Design review of the part built by this model. Coordinates are the model's own, in mm. A direction names the side the tool comes from. Coordinates: 2 decimals unless noted, no trailing zeros. Loops run counter-clockwise (first coordinate to the right, second up) from the corner with the lowest first, then second, coordinate; pieces in that order, holes last. Notation, with made-up numbers: (30, 16.5) - (85, 16.5) arc R13 ccw to (85, 25.5) - close; hole circle Ø7 at (48, 29). An arc over 180 degrees is marked (long way). Use one line per item in the form item = value. Start each with the question number.
(1) Add section D-D (z = 1.9). State the section outline as (x, y) points, plus the area to 3 significant figures.
(2) Add section B-B (z = 0.85). Count the separate pieces of the cut face and the enclosed holes in it, plus the area to 3 significant figures.
(3) The part is to be moulded in two halves that separate along Y. For faces 3 (the face through (-1, -0.29, 2)), 4 (the face through (0, 7.736, 1)), say which applies: pulls with the +Y half, pulls with the -Y half, needs draft (parallel to the pull), parting line crosses it, or undercut.
(4) Clearance check with flat-ended pins moving along their axes: pin 1 Ø1 at (x, z) = (-1.5, 2) entering from -Y; pin 2 Ø1.4 at (x, y) = (-2.53, 6.36) entering from +Z; pin 3 Ø2.5 at (x, y) = (-6.95, -1.31) entering from +Z. State where each tip first meets the part, or that it passes through.
(5) For L1, parallel to Y at x = 7, z = 0.6; L2, parallel to Y at x = -2.5, z = 0.75; L3, parallel to Y at x = -2.75, z = 1.3, list the stretches that pass through material, from the lowest coordinate up.
(6) Tool access review of faces 1 (the face through (-2.2, 1, 2)), 2 (the face through (-8.65, 7.45, 0.81)): name each direction out of +Z, -Z, +X, -X, +Y, -Y from which nothing blocks a thin tool from reaching the whole face with its end or side.
(7) Add section C-C (y = -1). State the section outline as (x, z) points, plus the area to 3 significant figures.
Autodesk Fusion 360 part; units mm, degrees
sketch "Sketch2" plane through (0, 0, 0) normal (0, 0, 1) x (1, 0, 0)
  line L0 (-8.9478, 7.7363) -> (9.0022, 7.7363)
  line L1 (9.0022, 7.7363) -> (9.0022, -5.5137)
  line L2 (9.0022, -5.5137) -> (-8.9478, -5.5137)
  line L3 (-8.9478, -5.5137) -> (-8.9478, 7.7363)
  line L4 (-8.9478, 7.7363) -> (9.0022, -5.5137) construction
  line L5 (-8.9478, -5.5137) -> (9.0022, 7.7363) construction
  line L6 (-9.5685, 6.7363) -> (10, 6.7363) construction
  line L7 (-9.5685, 6.3613) -> (10, 6.3613) construction
  line L8 (-10.5, -4.5137) -> (10.5, -4.5137) construction
  line L9 (-10.5, -4.1387) -> (10.5, -4.1387) construction
  line L10 (8.5022, 9) -> (8.5022, -6.5) construction
  line L11 (7.0022, 9) -> (7.0022, -6.5) construction
  line L12 (-8.4478, 9.5) -> (-8.4478, -7) construction
  line L13 (-6.9478, 9.5) -> (-6.9478, -7) construction
  line L14 (-10.5, -2.8137) -> (11.6299, -2.8137) construction
  line L15 (-10.5, -1.3137) -> (11.6299, -1.3137) construction
  circle A0 centre (7.0022, -1.3137) radius 1.5
  circle A1 centre (-6.9478, -1.3137) radius 1.5
  line L16 (-8.0478, 9) -> (-8.0478, 5) construction
  line L17 (-7.6728, 9) -> (-7.6728, 5) construction
  circle A2 centre (-7.6728, 6.3613) radius 0.375
  line L18 (-5.1028, 7.3) -> (-5.1028, 4.898) construction
  circle A3 centre (-5.1028, 6.3613) radius 0.375
  circle A4 centre (-2.5328, 6.3613) radius 0.375
  circle A5 centre (0.0372, 6.3613) radius 0.375
  circle A6 centre (2.5972, 6.3613) radius 0.375
  circle A7 centre (5.1672, 6.3613) radius 0.375
  circle A8 centre (7.7272, 6.3613) radius 0.375
  circle A9 centre (-7.6728, 6.3613) radius 0.875
  line L19 (-5.5478, -3.163) -> (-5.5478, -6) construction
  line L20 (-5.1728, -3.163) -> (-5.1728, -6) construction
  circle A10 centre (-5.1728, -4.1387) radius 0.375
  line L21 (-2.1478, -3.7) -> (-2.1478, -5.9) construction
  circle A11 centre (-2.5228, -4.1387) radius 0.375
  line L22 (-2.8978, -3.7) -> (-2.8978, -5.1) construction
  line L23 (0.4022, -3.6) -> (0.4022, -5.1) construction
  circle A12 centre (0.0272, -4.1387) radius 0.375
  line L24 (-0.3478, -3.6) -> (-0.3478, -5.3) construction
  circle A13 centre (2.5772, -4.1387) radius 0.375
  circle A14 centre (5.1272, -4.1387) radius 0.375
  line L25 (2.2022, -3.6) -> (2.2022, -5.1) construction
  line L26 (4.7522, -3.7) -> (4.7522, -5.1) construction
  line L27 (2.9522, -3.8) -> (2.9522, -4.9) construction
  line L28 (5.5022, -3.7) -> (5.5022, -5.1) construction
  circle A15 centre (-5.1028, 6.3613) radius 0.875
  circle A16 centre (-2.5328, 6.3613) radius 0.875
  circle A17 centre (0.0372, 6.3613) radius 0.875
  circle A18 centre (2.5972, 6.3613) radius 0.875
  circle A19 centre (5.1672, 6.3613) radius 0.875
  circle A20 centre (7.7272, 6.3613) radius 0.875
  circle A21 centre (5.1272, -4.1387) radius 0.875
  circle A22 centre (2.5772, -4.1387) radius 0.875
  circle A23 centre (0.0272, -4.1387) radius 0.875
  circle A24 centre (-2.5228, -4.1387) radius 0.875
  circle A25 centre (-5.1728, -4.1387) radius 0.875
  line L29 (-2.2, 2.4) -> (0.9, 2.4)
  line L30 (0.9, 2.4) -> (0.9, -0.2901)
  line L31 (0.9, -0.2901) -> (-2.2, -0.2901)
  line L32 (-2.2, -0.2901) -> (-2.2, 2.4)
  dimension "d1" = 17.95
  dimension "d2" = 13.25
  dimension "d3" = 1
  dimension "d4" = 0.375
  dimension "d5" = 1
  dimension "d6" = -0.375
  dimension "d7" = 0.5
  dimension "d8" = 1.5
  dimension "d9" = 0.5
  dimension "d10" = -1.5
  dimension "d11" = 2.7
  dimension "d12" = -1.5
  dimension "d13" = 3
  dimension "d14" = 3
  dimension "d15" = 0.9
  dimension "d17" = 0.75
  dimension "d19" = 2.57
  dimension "d21" = 0.75
  dimension "d22" = 0.75
  dimension "d23" = 2.57
  dimension "d24" = 0.75
  dimension "d25" = 2.57
  dimension "d26" = 0.75
  dimension "d27" = 2.56
  dimension "d28" = 0.75
  dimension "d29" = 2.57
  dimension "d30" = 0.75
  dimension "d31" = 2.56
  dimension "d32" = 0.5
  dimension "d33" = 3.4
  dimension "d34" = -0.375
  dimension "d35" = 0.75
  dimension "d36" = 3.4
  dimension "d37" = 0.75
  dimension "d38" = 0.75
  dimension "d39" = 3.3
  dimension "d40" = 0.75
  dimension "d41" = 0.75
  dimension "d42" = 3.3
  dimension "d43" = 3.3
  dimension "d44" = 0.5
  dimension "d45" = 0.5
  dimension "d46" = 0.5
  dimension "d47" = 0.5
  dimension "d48" = 0.5
  dimension "d49" = 0.5
  dimension "d50" = 0.5
  dimension "d51" = 0.5
  dimension "d52" = 0.5
  dimension "d53" = 0.5
  dimension "d54" = 0.5
extrude "Extrude1" add sketch "Sketch2" along normal blind 1.6 contours L0 L1 L2 L3 | A9 | A15 | A16 | A17 | A18 | A19 | A20 | A21 | A22 | A23 | A24 | A25 | L29 L30 L31 L32
extrude "Extrude2" add sketch "Sketch2" along normal blind 2.5 contours L29 L30 L31 L32
fillet "Fillet1" radius 1 4 edges at (-8.9478, -5.5137, 0.8) (9.0022, -5.5137, 0.8) (9.0022, 7.7363, 0.8) (-8.9478, 7.7363, 0.8)
sketch "Sketch3" plane through (0, 0, 1.6) normal (0, 0, 1) x (-1, 0, 0)
  line L0 (2.2, 0.2901) -> (2.2, -2.4)
  line L1 (2.2, -2.4) -> (-0.9, -2.4)
  line L2 (-0.9, -2.4) -> (-0.9, 0.2901)
  line L3 (-0.9, 0.2901) -> (2.2, 0.2901)
  circle A0 centre (-2.5972, -6.3613) radius 0.375
  circle A1 centre (-5.1272, 4.1387) radius 0.375
  circle A2 centre (-7.7272, -6.3613) radius 0.375
  circle A3 centre (5.1728, 4.1387) radius 0.375
  circle A4 centre (2.5228, 4.1387) radius 0.375
  circle A5 centre (-5.1672, -6.3613) radius 0.375
  circle A6 centre (-0.0272, 4.1387) radius 0.375
  circle A7 centre (-2.5772, 4.1387) radius 0.375
  circle A8 centre (-0.0372, -6.3613) radius 0.375
  circle A9 centre (2.5328, -6.3613) radius 0.375
  circle A10 centre (7.6728, -6.3613) radius 0.375
  circle A11 centre (6.9478, 1.3137) radius 1.5
  circle A12 centre (5.1028, -6.3613) radius 0.375
  circle A13 centre (-7.0022, 1.3137) radius 1.5
  arc A14 (7.9478, -7.7363) -> (8.9478, -6.7363) centre (7.9478, -6.7363) ccw
  line L4 (8.9478, -6.7363) -> (8.9478, 4.5137)
  arc A15 (8.9478, 4.5137) -> (7.9478, 5.5137) centre (7.9478, 4.5137) ccw
  line L5 (7.9478, 5.5137) -> (-8.0022, 5.5137)
  arc A16 (-8.0022, 5.5137) -> (-9.0022, 4.5137) centre (-8.0022, 4.5137) ccw
  line L6 (-9.0022, 4.5137) -> (-9.0022, -6.7363)
  arc A17 (-9.0022, -6.7363) -> (-8.0022, -7.7363) centre (-8.0022, -6.7363) ccw
  line L7 (-8.0022, -7.7363) -> (7.9478, -7.7363)
  circle A18 centre (-7.7272, -6.3613) radius 0.875
  circle A19 centre (-5.1672, -6.3613) radius 0.875
  circle A20 centre (-2.5972, -6.3613) radius 0.875
  circle A21 centre (-0.0372, -6.3613) radius 0.875
  circle A22 centre (2.5328, -6.3613) radius 0.875
  circle A23 centre (5.1028, -6.3613) radius 0.875
  circle A24 centre (7.6728, -6.3613) radius 0.875
  circle A25 centre (5.1728, 4.1387) radius 0.875
  circle A26 centre (2.5228, 4.1387) radius 0.875
  circle A27 centre (-0.0272, 4.1387) radius 0.875
  circle A28 centre (-2.5772, 4.1387) radius 0.875
  circle A29 centre (-5.1272, 4.1387) radius 0.875
extrude "Extrude3" cut sketch "Sketch3" against normal blind 0.01 contours A18 | A19 | A20 | A21 | A22 | A23 | A24 | A25 | A26 | A27 | A28 | A29
Computed values:
q1.outline = (-2.2, -0.29) - (0.9, -0.29) - (0.9, 2.4) - (-2.2, 2.4) - close
q1.area = 8.34 mm^2
q2.separate_pieces = 1
q2.enclosed_holes = 14
q2.area = 218 mm^2
q3.face_3 = pulls with the -Y half
q3.face_4 = pulls with the +Y half
q4.pin_1 = -5.51
q4.pin_2 = 1.59
q4.pin_3 = through
q5.L1 = -5.51 to -2.81, 0.19 to 7.74
q5.L2 = -5.51 to -4.51, -3.76 to 5.99, 6.73 to 7.74
q5.L3 = -5.51 to -4.44, -3.84 to 6.06, 6.67 to 7.74
q6.face_1 = +Z, -X, +Y, -Y
q6.face_2 = +Z, -Z, -X, +Y
q7.outline = (-8.95, 0) - (-8.41, 0) - (-8.41, 1.6) - (-8.95, 1.6) - close; (-5.48, 0) - (5.54, 0) - (5.54, 1.6) - (-5.48, 1.6) - close; (8.47, 0) - (9, 0) - (9, 1.6) - (8.47, 1.6) - close
q7.area = 19.3 mm^2
